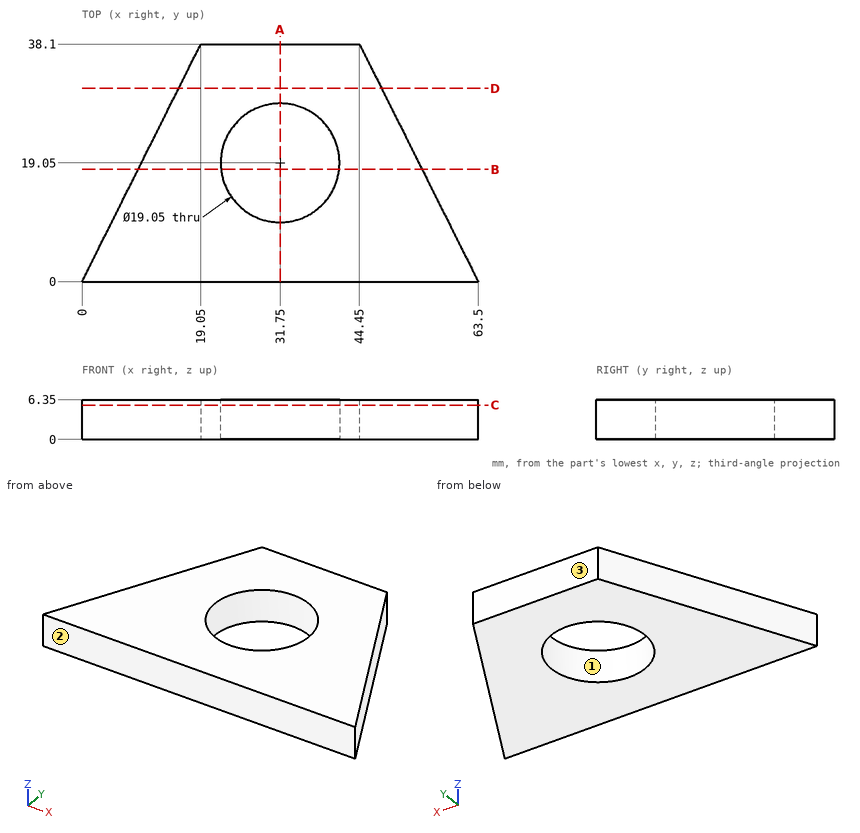
Answer from the drawing. Dimensions are ordinates in mm from the lowest x, y and z of the part. Round coordinates to 2 decimals unless told otherwise and drop trailing zeros. Loops run counter-clockwise (first coordinate to the right, second up) from the corner with the lowest first, then second, coordinate; pieces in that order, holes last.
1) Given P1, Ø1, axis at y = 21, z = 3, coming from the +X side; P2, Ø2, axis at y = 9.5, z = 3, coming from the -X side; P3, Ø22, axis at x = 31.75, y = 19.05, coming from the +Z side; P4, Ø1.5, axis at y = 33, z = 5.5, coming from the +X side (3 decimals), each flat-ended and moving along its own axis, determine where each tip first touches the part or whether it passes through.
Outcome:
P1: stops at x = 53.25
P2: stops at x = 4.25
P3: stops at z = 6.35
P4: stops at x = 47.375
2) For a pull along Y with two mould halves and no side action, classify the marked faces 1, 2 and 3 as released by +Y, released by -Y, zero draft, split by the parting line, or undercut.
Outcome:
face 1: undercut
face 2: released by -Y
face 3: released by +Y
3) A cutting plane is placed at D-D on y = 31. Determine the outline of the cut face in (x, z), plus the area to 3 significant figures.
Outcome:
outline: (15.5, 0) - (48, 0) - (48, 6.35) - (15.5, 6.35) - close
area: 206 mm2
4) A cutting plane is placed at A-A on x = 31.75. Determine the outline of the cut face in (y, z) (3 decimals), plus the area to 3 significant figures.
Outcome:
outline: (0, 0) - (9.525, 0) - (9.525, 6.35) - (0, 6.35) - close; (28.575, 0) - (38.1, 0) - (38.1, 6.35) - (28.575, 6.35) - close
area: 121 mm2
5) Consider line 1 (Y direction, x = 31.75, z = 4.5) (3 decimals); line 2 (Y direction, x = 33, z = 5.25); line 3 (X direction, y = 18, z = 5.75). Determine where each line is inside the solid, lowest interval first.
Outcome:
line 1: y = 0 to 9.525, 28.575 to 38.1
line 2: y = 0 to 9.61, 28.49 to 38.1
line 3: x = 9 to 22.28, 41.22 to 54.5
6) A cutting plane is placed at B-B on y = 18. Determine the outline of the cut face in (x, z), plus the area to 3 significant figures.
Outcome:
outline: (9, 0) - (22.28, 0) - (22.28, 6.35) - (9, 6.35) - close; (41.22, 0) - (54.5, 0) - (54.5, 6.35) - (41.22, 6.35) - close
area: 169 mm2
7) A cutting plane is placed at C-C on z = 5.5. Determine the outline of the cut face in (x, y) (3 decimals), plus the area to 3 significant figures.
Outcome:
outline: (0, 0) - (63.5, 0) - (44.45, 38.1) - (19.05, 38.1) - close; hole circle Ø19.05 at (31.75, 19.05)
area: 1,410 mm2
